Source: CAD feature listing. Evaluate the final solid. Frame: model axes, mm. Face numbers are marked on the shaded views. A direction names the side the tool comes from. Coordinates: 2 decimals unless noted, no trailing zeros. Write each loop counter-clockwise with the first axis right and the second up, starting at its lowest first coordinate (ties: lowest second). Pieces come first, ordered by that corner, then holes. Notation, with made-up numbers: M 89.5,85.5 L 111.5,85.5 A32 ccw 111.5,119.5 Z; hole C 2.25,77.5 d10. An arc over 180 degrees is marked long. One line per item, written item: value. Start each with the question number.
Item 1: Ray query, L1, parallel to Y at x = 0, z = 8.55; L2, parallel to Y at x = 1.5, z = 5.5. Return the intervals inside material, ascending. Write a range as from..to.
Item 2: Set-up query: the marked faces 1, 2, 3 and 4. Return all of +Z, -Z, +X, -X, +Y, -Y with unobstructed straight access to the full face (end or side cutting, diameter ignored); none if empty.
Item 3: Cut plane C-C, the plane y = 13. Output: boundary loops of the cut face in (x, z), then the cut area to 3 significant figures.
Item 4: Cut plane D-D, the plane x = -1. Output: boundary loops of the cut face in (y, z).
Item 5: Pin query (flat end, axial travel): P1, Ø1.5, axis at x = 1.5, z = 8.5, coming from the +Y side; P2, Ø0.8, axis at y = -1, z = 9, coming from the -X side; P3, Ø3, axis at y = 19.5, z = 3, coming from the +X side. Return the tip coordinate at first contact, or that it passes through.
Item 6: Cut plane B-B, the plane z = 5.5. Output: boundary loops of the cut face in (x, y).
Item 7: Cut plane A-A, the plane x = 13.5. Output: boundary loops of the cut face in (y, z).
Item 8: Mould query, pull axis X, two halves, no side actions, for the marked faces 5, 6, 7 and 8. Classes: released by +X, released by -X, zero draft, split by the parting line, or undercut.
```python
from build123d import *

# Parameters (mm, degrees)
SKETCH003_W   = 12.468703
SKETCH003_H   = 5.180136
SKETCH003_W_2 = 5.180136
SKETCH003_H_2 = 12.468704
PAD003_DEPTH  = 5
SKETCH002_R   = 4
PAD002_DEPTH  = 18
SKETCH001_R   = 4
PAD001_DEPTH  = 18
PAD005_DEPTH  = 7
SKETCH004_W   = 4
SKETCH004_H   = 2
SKETCH004_W_2 = 2
SKETCH004_H_2 = 4
PAD004_DEPTH  = 2.5
SKETCH_R      = 4
PAD_DEPTH     = 10


with BuildPart() as nutmount:
    # Sketch003 → Pad003 (new body)
    with BuildSketch(Plane.XY.offset(10)):
        with Locations((-1.285158, 14.590068)):
            Rectangle(SKETCH003_W, SKETCH003_H)
        with Locations((14.590068, -0.774081)):
            Rectangle(SKETCH003_W_2, SKETCH003_H_2)
    extrude(amount=-PAD003_DEPTH)


with BuildPart() as mount002:
    # Sketch002 → Pad002 (new body)
    with BuildSketch(Plane.XZ.offset(-27)):
        with Locations((-1, 10)):
            Circle(SKETCH002_R)
    extrude(amount=PAD002_DEPTH)


with BuildPart() as mount001:
    # Sketch001 → Pad001 (new body)
    with BuildSketch(Plane.YZ.offset(27)):
        with Locations((-1, 10)):
            Circle(SKETCH001_R)
    extrude(amount=-PAD001_DEPTH)


with BuildPart() as obj1:
    # Sketch005 → Pad005 (new body)
    with BuildSketch(Plane(origin=(0, 0, 0), x_dir=(1, 0, 0), z_dir=(0, 0, -1))):
        Polygon((3.65, -6.321985), (7.3, 0), (3.65, 6.321985), (-3.65, 6.321985), (-7.3, 0), (-3.65, -6.321985), align=None)
    extrude(amount=-PAD005_DEPTH)


with BuildPart() as cutblock:
    # Sketch004 → Pad004 (new body)
    with BuildSketch(Plane.XY.offset(10)):
        with Locations((0, 6.5)):
            Rectangle(SKETCH004_W, SKETCH004_H)
        with Locations((6.5, 0)):
            Rectangle(SKETCH004_W_2, SKETCH004_H_2)
        Polygon((-6.717514, -3.889087), (-5.303301, -2.474874), (-2.474874, -5.303301), (-3.889087, -6.717514), align=None)
    extrude(amount=-PAD004_DEPTH)

    # Fusion: union NutMount, Mount002, Mount001, obj1
    add(nutmount.part)
    add(mount002.part)
    add(mount001.part)
    add(obj1.part)


with BuildPart() as cut:
    # Sketch → Pad (new body)
    with BuildSketch(Plane.XY):
        with BuildLine():
            Line((-9, 3.6e-05), (-9, 27))
            Line((-9, 27), (7, 27))
            Line((7, 27), (7, 7))
            Line((7, 7), (27, 7))
            Line((27, 7), (27, -9))
            Line((27, -9), (3.6e-05, -9))
            ThreePointArc((-9, 3.6e-05), (-6.363961, -6.363961), (3.6e-05, -9))
        make_face()
        Circle(SKETCH_R, mode=Mode.SUBTRACT)
    extrude(amount=PAD_DEPTH)

    # Cut: cut CutBlock
    add(cutblock.part, mode=Mode.SUBTRACT)


solid = cut.part
```
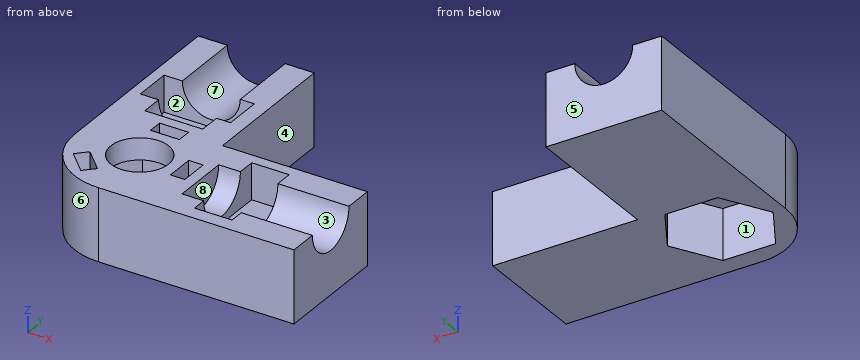
From the geometry:
1. L1: y = -9..-4, 4..5.5, 7.5..9
1. L2: y = -9..-6.32, 6.32..12, 17.18..27
2. face 1: -Z
2. face 2: +Z
2. face 3: +Z, +X
2. face 4: +Z, -Z, +X, +Y
3. outline: M -9,0 L 7,0 L 7,10 L 4.95,10 L 4.95,5 L -7.52,5 L -7.52,10 L -9,10 Z
3. area: 97.7 mm²
4. outline: M -8.94,0 L -6.32,0 L -6.32,7 L -3.87,7 L -3.87,10 L -8.94,10 Z; M 3.87,7 L 6.32,7 L 6.32,0 L 27,0 L 27,6 L 17.18,6 L 17.18,5 L 12,5 L 12,6 L 9,6 L 9,10 L 7.5,10 L 7.5,7.5 L 5.5,7.5 L 5.5,10 L 3.87,10 Z
5. P1: stops at y = 9
5. P2: stops at x = -8.98
5. P3: stops at x = 7
6. outline: M -9,0 A9 ccw 0,-9 L 27,-9 L 27,7 L 7,7 L 7,27 L -9,27 Z; hole M -7.52,12 L 4.95,12 L 4.95,17.18 L -7.52,17.18 Z; hole M -7.3,0 L -3.65,-6.32 L 3.65,-6.32 L 7.3,0 L 3.65,6.32 L -3.65,6.32 Z; hole M 12,-7.01 L 17.18,-7.01 L 17.18,5.46 L 12,5.46 Z
7. outline: M -9,0 L 7,0 L 7,10 L 5.46,10 L 5.46,5 L -7.01,5 L -7.01,10 L -9,10 Z
8. face 5: zero draft
8. face 6: released by -X
8. face 7: undercut
8. face 8: released by +X
